Part model, mm, in its own coordinate system. A direction names the side the tool comes from. Give positions to 0.01 mm unless a question says otherwise; leave off trailing zeros. Order: outer loops, then holes, each group sorted by start corner. A loop starts at its lowest first (then second) coordinate and runs counter-clockwise, first axis right, second up. Notation, with made-up numbers: (14.5, 22) -> (62.5, 22) arc R27 cw to (62.5, 41) -> close; hole circle Ø5 at (33.5, 52.25). An arc over 180 degrees is marked (long way). Write item = value, one per line. Start each with the question number.
Item 1: Pull direction Y, two halves, no side cores. Call faces 1 (the face through (46.208, 28.827, -5.601)), 2 (the face through (20, 37.5, 0)), 3 (the face through (20, 0, 0)): +Y half, -Y half, draft (parallel to the pull), parting line (faces both ways), or undercut.
Item 2: Drill centre lines: line 1 along X through (y, z) = (27.95, -5); line 2 along Z through (x, y) = (44.3, 28.9); line 3 along Y through (x, z) = (23, 1). Where is each one in solid material? Low to high.
Item 3: Band-saw the part on C-C on x = 30. Write the cut outline in (y, z), plus the area to 3 significant figures.
Item 4: Tool access for faces 4 (the face through (26.515, 44.31, 4.625)), 5 (the face through (0, 14, 0)), 6 (the face through (20, 19, 10)), 7 (the face through (20, 19, -10)): list every direction of +Z, -Z, +X, -X, +Y, -Y with a clear straight run to the whole face (end or side of a thin tool).
Item 5: Flat gauge pins, fed straight in: P1, Ø5.5, axis at y = 34.5, z = 5, coming from the -X side; P2, Ø2, axis at x = -3, z = 3.5, coming from the +Y side; P3, Ø2, axis at y = 33, z = 5, coming from the +X side. Where does each tip first touch, or does it go through?
Item 6: Band-saw the part on A-A on x = -4.3. Write the cut outline in (y, z).
Item 7: Band-saw the part on B-B on z = -5. Count the separate pieces of the cut face and the enclosed holes in it, plus the area to 3 significant figures.
Item 8: Band-saw the part on D-D on z = 0. Write the cut outline in (x, y), plus the area to 3 significant figures.
Autodesk Inventor part; units mm, degrees
ref_plane "YZ Plane" through (0, 0, 0) normal (1, 0, 0) x (0, 1, 0)
ref_plane "XZ Plane" through (0, 0, 0) normal (0, 1, 0) x (-1, 0, 0)
ref_plane "XY Plane" through (0, 0, 0) normal (0, 0, 1) x (1, 0, 0)
sketch "草圖1" plane through (0, 0, 0) normal (0, 0, 1) x (1, 0, 0)
  line L0 (0, 0) -> (40, 0)
  line L1 (40, 0) -> (40, 37.5)
  line L2 (40, 37.5) -> (0, 37.5)
  line L3 (0, 37.5) -> (0, 0)
  dimension "d0" = 37.5
  dimension "d1" = 40
extrude "擠出1" add sketch "草圖1" along normal mid plane 20
sketch "草圖2" plane through (0, 0, 10) normal (0, 0, 1) x (1, 0, 0)
  line L0 (-7, 31.9) -> (47, 31.9)
  line L1 (47, 31.9) -> (47, 26.9)
  line L2 (47, 26.9) -> (-7, 26.9)
  line L3 (-7, 26.9) -> (-7, 31.9)
  line L4 (0, 37.5) -> (0, 0)
  line L5 (0, 0) -> (40, 0)
  dimension "d4" = 54
  dimension "d5" = 7
  dimension "d6" = 26.9
  dimension "d7" = 5
extrude "擠出2" add sketch "草圖2" against normal blind 20
sketch "草圖3" plane through (-7, 31.9, 10) normal (0, 1, 0) x (1, 0, 0)
  line L0 (2.7, 15) -> (51.3, 15)
  line L1 (51.3, 15) -> (51.3, 5)
  line L2 (51.3, 5) -> (2.7, 5)
  line L3 (2.7, 5) -> (2.7, 15)
  line L4 (47, 20) -> (54, 20)
  line L5 (54, 0) -> (54, 20)
  circle A0 centre (2.7, 15) radius 2
  circle A1 centre (2.7, 5) radius 2
  circle A2 centre (51.3, 5) radius 2
  circle A3 centre (51.3, 15) radius 2
  point P0 (7, 10)
  dimension "d10" = 10
  dimension "d11" = 5
  dimension "d12" = 2.7
  dimension "d13" = 48.6
  dimension "d14" = 4
extrude "擠出3" cut sketch "草圖3" against normal blind 20 contours L3 A0 L0 | L0 A0 L3 | A3 L1 L0 | L0 L1 A3 | A1 L2 L3 | L3 L2 A1 | A2 L2 L1 | L1 L2 A2
sketch "草圖4" plane through (0, 0, 0) normal (0, 0, 1) x (1, 0, 0)
  line L0 (0, 37.5) -> (40, 37.5)
  line L1 (32, 37.5) -> (30, 37.5)
  line L2 (30, 37.5) -> (30, 45.7)
  line L3 (30, 45.7) -> (32, 45.7)
  line L4 (32, 45.7) -> (32, 37.5)
  line L5 (-2.3, 26.9) -> (-6.3, 26.9)
  line L6 (-6.3, 31.9) -> (-2.3, 31.9)
  line L7 (-4.3, 26.9) -> (-4.3, 31.9)
  line L8 (40, 0) -> (0, 0)
  line L9 (30, 45.7) -> (40.2, 45.7)
  line L10 (40.2, 45.7) -> (40.2, 42.9583)
  line L11 (40.2, 42.9583) -> (30, 42.9583)
  line L12 (30, 42.9583) -> (30, 45.7)
  dimension "d17" = 34.3
  dimension "d18" = 45.7
  dimension "d19" = 2
  dimension "d20" = 10.2
revolve "迴轉1" add sketch "草圖4" angle 360 about axis through (30, 37.5, 0) along (0, 1, 0)
sketch "草圖5" plane through (30, 45.7, 0) normal (0, 1, 0) x (1, 0, 0)
  line L0 (-4.9497, -4.9497) -> (4.9497, -4.9497)
  line L1 (4.9497, -4.9497) -> (4.9497, 4.9497)
  line L2 (4.9497, 4.9497) -> (-4.9497, 4.9497)
  line L3 (-4.9497, 4.9497) -> (-4.9497, -4.9497)
  line L4 (-4.9497, -4.9497) -> (4.9497, 4.9497) construction
  line L5 (4.9497, -4.9497) -> (-4.9497, 4.9497) construction
  circle A0 centre (0, 0) radius 10.2
  point P0 (-30, 0)
  point P1 (0, 0)
  dimension "d22" = 14
hole "孔1" at (34.9497, 45.7, -4.9497) at (34.9497, 45.7, 4.9497) at (25.0503, 45.7, 4.9497) at (25.0503, 45.7, -4.9497) direction (0, -1, 0) diameter 3 depth 4 tip angle 118
move faces "移動1" translate (0, -1.2, 0) faces at (-0.786, 31.9, -1.5071)
move faces "移動2" translate (0, -1.2, 0) faces at (40.786, 31.9, 1.5071)
properties part number "MG996 伺服馬達"
Values found:
q1.face_1 = draft
q1.face_2 = undercut
q1.face_3 = -Y half
q2.line_1 = -7 to -6.3, -2.3 to 42.3, 46.3 to 47
q2.line_2 = -10 to -7, -3 to 3, 7 to 10
q2.line_3 = 0 to 37.5, 42.96 to 45.7
q3.outline = (0, -10) -> (37.5, -10) -> (37.5, -2) -> (42.96, -2) -> (42.96, -10.2) -> (45.7, -10.2) -> (45.7, 10.2) -> (42.96, 10.2) -> (42.96, 2) -> (37.5, 2) -> (37.5, 10) -> (0, 10) -> close
q3.area = 828 mm^2
q4.face_4 = +Y
q4.face_5 = +Z, -Z, -X, -Y
q4.face_6 = +Z, +X, -X, -Y
q4.face_7 = -Z, +X, -X, -Y
q5.P1 = 0
q5.P2 = 30.7
q5.P3 = 40
q6.outline = (26.9, -10) -> (30.7, -10) -> (30.7, -7) -> (26.9, -7) -> close; (26.9, -3) -> (30.7, -3) -> (30.7, 3) -> (26.9, 3) -> close; (26.9, 7) -> (30.7, 7) -> (30.7, 10) -> (26.9, 10) -> close
q7.separate_pieces = 6
q7.enclosed_holes = 0
q7.area = 1,560 mm^2
q8.outline = (-7, 26.9) -> (0, 26.9) -> (0, 0) -> (40, 0) -> (40, 26.9) -> (47, 26.9) -> (47, 30.7) -> (40, 30.7) -> (40, 37.5) -> (32, 37.5) -> (32, 42.96) -> (40.2, 42.96) -> (40.2, 45.7) -> (19.8, 45.7) -> (19.8, 42.96) -> (28, 42.96) -> (28, 37.5) -> (0, 37.5) -> (0, 30.7) -> (-7, 30.7) -> close
q8.area = 1,630 mm^2
